```python
from build123d import *

# Parameters (mm, degrees)
F2_DEPTH = 5
F3_DEPTH = 5
F5_COUNT = 10
F5_ANGLE = 324


with BuildPart() as f2:
    # F1 (on Front) → F2 (new body)
    with BuildSketch(Plane.XZ):
        with BuildLine():
            ThreePointArc((7.9991114538, -0.1192306565), (7.9997778604, -0.0596169837), (8, 0))
            ThreePointArc((8, 0), (7.8460497183, 1.5618911033), (7.3901240454, 3.0636688127))
            ThreePointArc((7.3901240454, 3.0636688127), (-7.857471258, -1.5033780063), (7.9991114538, -0.1192306565))
        make_face()
    extrude(amount=F2_DEPTH)

    # F1 (on Front) → F3 (join)
    with BuildSketch(Plane.XZ):
        with BuildLine():
            ThreePointArc((7.3901240454, 3.0636688127), (7.8460497183, 1.5618911033), (8, 0))
            ThreePointArc((8, 0), (7.9997778604, -0.0596169837), (7.9991114538, -0.1192306565))
            ThreePointArc((7.9991114538, -0.1192306565), (9.3543332011, 0.3818427302), (10.4105264675, 1.3678226019))
            ThreePointArc((10.4105264675, 1.3678226019), (10.3129310261, 1.9731836333), (10.180165277, 2.5718154938))
            ThreePointArc((10.180165277, 2.5718154938), (8.8345975473, 3.0982639794), (7.3901240454, 3.0636688127))
        make_face()
    extrude(amount=F3_DEPTH)

    # F5: F2 ×10 about axis
    f5_axis = Axis((0, 6.1465417966, 0), (0, 1, 0))


with BuildPart() as f2_1:
    add(f2.part)
    for i in range(1, F5_COUNT):
        add(f2.part.rotate(f5_axis, i * F5_ANGLE / (F5_COUNT - 1)))


solid = f2_1.part
```
Could you check a few things on this model? Use its own coordinates, in mm. A direction names the side the tool comes from. Coordinates: 2 decimals unless noted, no trailing zeros. Loops run counter-clockwise (first coordinate to the right, second up) from the corner with the lowest first, then second, coordinate; pieces in that order, holes last. Notation, with made-up numbers: M -31,-22 L 8,-22 A33 cw 8,13 Z; hole C 53,81 d11. An arc over 180 degrees is marked long. Put each result on its own line as item: value. Start each with the question number.
(1) Suppose I cut it at A-A on x = 8.25. Please give me the cut outline in (y, z), then the cut area to 3 significant figures.
(2) I need wall thicknesses on line 1 (X direction, y = -1.1, z = -8.25); line 2 (X direction, y = -3.85, z = -8.5); line 3 (X direction, y = -3.55, z = -0.25). Which ranges of each line are inside material? Lowest first, please. Write a range as from..to.
(3) For faces 1 (the face through (-0.207, -2.465, 9.378)), 2 (the face through (2.532, -2.465, 8.995)), 3 (the face through (-7.936, -2.465, 1.011)), 4 (the face through (-5.345, -2.465, -7.708)), 5 (the face through (7.336, -2.465, 5.788)), which set-ups out of +Z, -Z, +X, -X, +Y, -Y let a thin tool reach every point of the face, with its end or its side?
(4) Will these pins go through, and if not, where does the flat tip stop? P1, Ø3, axis at y = -1, z = -3, coming from the +X side; P2, Ø6, axis at x = -2, z = -8.5, coming from the +Y side; P3, Ø1.5, axis at x = -1.5, y = -3, coming from the -Z side; P4, Ø3, axis at x = 4, y = -3.5, coming from the -Z side.
(5) Suppose I cut it at B-B on z = -1. Please give me the cut outline in (x, y).
(6) Suppose I cut it at C-C on x = -1.5. Please give me the cut outline in (y, z), then the cut area to 3 significant figures.
(7) Thinking about a two-plate mould opening in Z: for faces 6 (the face through (7.19, -2.46, 7.65)), 7 (the face through (5.68, -2.46, -7.46)), 8 (the face through (-10.315, -2.465, -1.965)), which applies, pulls with the +Z half, pulls with the -Z half, needs draft (parallel to the pull), parting line crosses it, or undercut?
Solutions:
1. outline: M -5,-5.2 L 0,-5.2 L 0,-2.11 L -5,-2.11 Z; M -5,-0.07 L 0,-0.07 L 0,3.15 L -5,3.15 Z
1. area: 31.6 mm2
2. line 1: x = -2.63..0.59, 2.74..5.7
2. line 2: x = -2.61..0.54, 2.96..5.67
2. line 3: x = -9.12..8
3. face 1: +Z, +Y, -Y
3. face 2: +Y, -Y
3. face 3: -X, +Y, -Y
3. face 4: -Z, +Y, -Y
3. face 5: +X, +Y, -Y
4. P1: stops at x = 9.75
4. P2: stops at y = 0
4. P3: stops at z = -10.47
4. P4: stops at z = -9.48
5. outline: M -10.11,-5 L 7.94,-5 L 7.94,0 L -10.11,0 Z
6. outline: M -5,-10.39 L 0,-10.39 L 0,7.86 L -5,7.86 Z
6. area: 91.3 mm2
7. face 6: pulls with the +Z half
7. face 7: undercut
7. face 8: pulls with the -Z half
